Autodesk Inventor part; units mm, degrees
ref_plane "YZ Plane" through (0, 0, 0) normal (1, 0, 0) x (0, 1, 0)
ref_plane "XZ Plane" through (0, 0, 0) normal (0, 1, 0) x (-1, 0, 0)
ref_plane "XY Plane" through (0, 0, 0) normal (0, 0, 1) x (1, 0, 0)
sketch "スケッチ1" plane through (0, 0, 0) normal (0, 1, 0) x (-1, 0, 0)
  circle A0 centre (0, 0) radius 178.1675
  circle A1 centre (0, 0) radius 157.8276
  line L0 (168.1877, 0) -> (166.7488, -21.9529)
  line L1 (168.1877, 0) -> (130.1721, 2.4917) construction
  line L2 (249.4344, 0) -> (-249.4344, 0)
  line L3 (166.7488, -21.9529) -> (156.7702, -21.2989)
  line L4 (156.7702, -21.2989) -> (158.2091, 0.654) construction
  line L5 (158.2091, 0.654) -> (168.1877, 0)
  line L6 (157.4896, -10.3224) -> (0, 0)
  line L7 (166.7488, -21.9529) -> (162.4568, -43.5302)
  line L8 (162.4568, -43.5302) -> (152.649, -41.5793) construction
  line L9 (152.649, -41.5793) -> (156.9409, -20.002) construction
  line L10 (156.9409, -20.002) -> (166.7488, -21.9529) construction
  line L11 (162.4568, -43.5302) -> (155.3851, -64.3626)
  line L12 (155.3851, -64.3626) -> (145.9158, -61.1482) construction
  line L13 (145.9158, -61.1482) -> (152.9875, -40.3158) construction
  line L14 (152.9875, -40.3158) -> (162.4568, -43.5302) construction
  line L15 (155.3851, -64.3626) -> (145.6548, -84.0938)
  line L16 (145.6548, -84.0938) -> (136.6861, -79.6709) construction
  line L17 (136.6861, -79.6709) -> (146.4164, -59.9397) construction
  line L18 (146.4164, -59.9397) -> (155.3851, -64.3626) construction
  line L19 (0, 0) -> (111.6009, -111.6009)
  line L20 (145.6548, -84.0938) -> (137.3401, -78.5381) construction
  line L21 (137.3401, -78.5381) -> (125.1176, -96.8305) construction
  line L22 (125.1176, -96.8305) -> (133.4323, -102.3862) construction
  line L23 (133.4323, -102.3862) -> (145.6548, -84.0938)
  line L24 (133.4323, -102.3862) -> (125.9139, -95.7927) construction
  line L25 (125.9139, -95.7927) -> (111.4082, -112.3332) construction
  line L26 (111.4082, -112.3332) -> (118.9266, -118.9266)
  line L27 (118.9266, -118.9266) -> (133.4323, -102.3862)
  line L28 (111.6009, -111.6009) -> (118.9266, -118.9266)
  line L29 (166.7488, -21.9529) -> (176.7274, -22.6069) construction
  line L30 (118.9266, -118.9266) -> (125.9834, -125.9834)
  point P0 (154.795, -30.7906)
  point P1 (149.4517, -50.732)
  point P2 (141.5512, -69.8053)
  point P3 (131.2288, -87.6843)
  point P4 (118.661, -104.0629)
  point P5 (157.8276, 0)
  point P6 (178.1675, 0)
  dimension "d0" = 22
  dimension "d1" = 10
  dimension "d2" = 45
  dimension "d4" = 315.6551
extrude "押し出し1" add sketch "スケッチ1" along normal blind 5.5 contours L30 L27 L23 L15 L11 L7 L0 L2 A0 | L28 A1 L2 L0 L7 L11 L15 L23 L27
sketch "スケッチ2" plane through (0, 5.5, 0) normal (0, 1, 0) x (1, 0, 0)
  circle A0 centre (0, 0) radius 309.8276
  line L0 (-168.1877, 0) -> (-166.7488, 21.9529)
  line L1 (-166.7488, 21.9529) -> (-162.4568, 43.5302)
  line L2 (-162.4568, 43.5302) -> (-155.3851, 64.3626)
  line L3 (-155.3851, 64.3626) -> (-145.6548, 84.0938)
  line L4 (-133.4323, 102.3862) -> (-145.6548, 84.0938)
  line L5 (-118.9266, 118.9266) -> (-133.4323, 102.3862)
  line L6 (-167.4682, 10.9764) -> (-166.0294, 32.9293)
  line L7 (-166.0294, 32.9293) -> (-275.7938, 40.1237)
  line L8 (-275.7938, 40.1237) -> (-277.2327, 18.1708)
  line L9 (-277.2327, 18.1708) -> (-167.4682, 10.9764)
  line L10 (-164.6028, 32.7415) -> (-160.3108, 54.3188)
  line L11 (-160.3108, 54.3188) -> (-268.1972, 75.7787)
  line L12 (-268.1972, 75.7787) -> (-272.4892, 54.2015)
  line L13 (-272.4892, 54.2015) -> (-164.6028, 32.7415)
  circle A1 centre (-166.7488, 21.9529) radius 11
  circle A2 centre (-162.4568, 43.5302) radius 11
  line L14 (-158.921, 53.9464) -> (-151.8493, 74.7789)
  line L15 (-151.8493, 74.7789) -> (-256.0116, 110.1372)
  line L16 (-256.0116, 110.1372) -> (-263.0833, 89.3047)
  line L17 (-263.0833, 89.3047) -> (-158.921, 53.9464)
  circle A3 centre (-155.3851, 64.3626) radius 11
  arc A4 (-275.7591, 62.4834) -> (-281.3553, 41.7349) centre (-166.7488, 21.9529) ccw
  line L18 (-178.1663, 0.654) -> (-158.2091, -0.654)
  line L19 (-158.2091, -0.654) -> (-156.7702, 21.2989)
  line L20 (-156.7702, 21.2989) -> (-176.7274, 22.6069)
  line L21 (-176.7274, 22.6069) -> (-178.1663, 0.654)
  line L22 (-177.4468, 11.6305) -> (-275.7938, 40.1237)
  line L23 (-176.7274, 22.6069) -> (-176.008, 33.5834)
  line L24 (-176.008, 33.5834) -> (-275.7591, 62.4834)
  line L25 (-275.7938, 40.1237) -> (-281.3553, 41.7349)
  circle A5 centre (0, 0) radius 137.8276
  line L26 (0, 0) -> (-219.0812, 219.0812)
  line L27 (-111.6009, 111.6009) -> (-125.9834, 125.9834)
  line L28 (-433.7586, 0) -> (433.7586, 0)
  circle A6 centre (0, 0) radius 279.8276 construction
  arc A7 (-111.6009, 111.6009) -> (-157.8276, 0) centre (0, 0) ccw
  point P0 (-158.1662, 0)
  point P1 (-137.8276, 0)
  point P2 (-97.4588, 97.4588)
  point P3 (-309.8276, 0)
  dimension "d7" = 22
  dimension "d10" = 20
  dimension "d11" = 100
  dimension "d12" = 30
  dimension "d14" = 20
  dimension "d17" = 122
extrude "押し出し2" add sketch "スケッチ2" against normal blind 5.5 contours L26 L5 L4 L3 A3 L15 L16 L17 A2 L11 L12 L24 A4 L25 L8 L9 L21 L18 L28 A0 | L18 L21 L9 L0 | L0 A1 L19 L28 | A5 L28 A7 A1 A2 A3 L26 | L26 A7 A3 L3 L4 L5 | A1 L21 L20 L0 | L9 L21 A1 | L0 L20 L19 A1 | L19 A7 L28 | L6 A1 L1 | L20 L23 A1 L6 | L1 A1 A7 L19 L20 | L22 L7 L23 A1 L21 | L9 L8 L22 | A1 L23 L21 | A1 A7 L19 | A7 A3 L2 L3 | A3 A7 | A2 L10 L1 | A1 L7 L24 L13 | A2 A7 A1 | L13 L24 L12 L11 A2 | L1 L2 A2 A7 | A1 L23 L7 | L25 A4 L24 L12 L13 L7 | A7 A1 | A7 A2 A3 | L3 L14 A3 | L10 A2 L2 | L13 L12 L24 | A7 A2 | A3 L14 L2 | L17 L16 L15 A3
sketch "スケッチ3" plane through (0, 5.5, 0) normal (0, 1, 0) x (1, 0, 0)
  circle A0 centre (0, 0) radius 157.8276
  arc A1 (-97.4588, 97.4588) -> (-137.8276, 0) centre (0, 0) ccw
  line L0 (-97.4588, 97.4588) -> (-219.0812, 219.0812)
  line L1 (-309.8276, 0) -> (-137.8276, 0)
  arc A2 (-219.0812, 219.0812) -> (-309.8276, 0) centre (0, 0) ccw
  point P0 (-157.8276, 0)
  point P1 (-111.6009, 111.6009)
  dimension "d18" = 20
extrude "押し出し3" cut sketch "スケッチ3" against normal through all contours A0 L1 A2 L0
sketch "スケッチ4" plane through (0, 5.5, 0) normal (0, 1, 0) x (1, 0, 0)
  arc A0 (-111.6009, 111.6009) -> (-157.8276, 0) centre (0, 0) ccw
  line L0 (-157.8276, 0) -> (-137.8276, 0)
  line L1 (-137.8276, 0) -> (-137.8276, 25)
  line L2 (-137.8276, 25) -> (-157.8276, 25)
  line L3 (-157.8276, 25) -> (-157.8276, 0)
  arc A1 (-97.4588, 97.4588) -> (-137.8276, 0) centre (0, 0) ccw
  line L4 (-97.4588, 97.4588) -> (-111.6009, 111.6009)
  line L5 (-111.6009, 111.6009) -> (-129.2786, 93.9233)
  line L6 (-129.2786, 93.9233) -> (-115.1365, 79.7811)
  line L7 (-115.1365, 79.7811) -> (-97.4588, 97.4588)
  dimension "d21" = 25
  dimension "d22" = 25
extrude "押し出し4" cut sketch "スケッチ4" against normal through all contours L4 L7 L6 A0 | A0 L6 L5 | L2 L1 L0 A0 | A0 L3 L2
fillet "フィレット1" radius 1 2 edges at (-97.4588, 2.75, -97.4588) (-137.8276, 2.75, 0)
sketch "スケッチ5" plane through (0, 5.5, 0) normal (0, 1, 0) x (1, 0, 0)
  circle A0 centre (0, 0) radius 147.8276
  arc A1 (-127.8696, 92.5143) -> (-155.835, 25) centre (0, 0) ccw
  arc A2 (-137.8276, 23.48) -> (-135.842, 23.3109) centre (-136.8276, 23.48) ccw
  arc A3 (-112.5381, 79.5715) -> (-135.842, 23.3109) centre (0, 0) ccw
  arc A4 (-112.5381, 79.5715) -> (-114.0617, 80.8559) centre (-113.3546, 80.1488) ccw
  line L0 (-114.0617, 80.8559) -> (-115.1365, 79.7811)
  line L1 (-115.1365, 79.7811) -> (-127.8696, 92.5143)
  arc A5 (-127.8696, 92.5143) -> (-155.835, 25) centre (0, 0) ccw
  line L2 (-155.835, 25) -> (-137.8276, 25)
  line L3 (-137.8276, 25) -> (-137.8276, 23.48)
  point P0 (-120.7019, 85.3466)
  point P1 (-145.6983, 25)
  dimension "d26" = 10
extrude "押し出し5" cut sketch "スケッチ5" against normal through all contours L1 L0 A4 A3 A2 L3 L2 A0 picked at (-137.0003, 45.2919)
equation "\"d22\" = d21"
properties part number "back_upper" material "木材 (カエデ材)"
Geometry: final body of the model. Coordinates: model frame, mm. Round coordinates to 2 decimals unless told otherwise and drop trailing zeros. Order: outer loops, then holes, each group sorted by start corner. A loop starts at its lowest first (then second) coordinate and runs counter-clockwise, first axis right, second up. Notation, with made-up numbers: (-0.5, -23.75) -> (43.5, -23.75) arc R38 cw to (43.5, 14.25) -> close; hole circle Ø9 at (-7, 43). An arc over 180 degrees is marked (long way). Put each result on its own line as item: value. Start each with the question number.
Q1. Line query: probe 1 along Z at (x, y) = (-137.5, 2.1); probe 2 along Z at (x, y) = (-123, 2); probe 3 along X at (y, z) = (2.3, -64.5). Output: solid intervals per line, ascending.
Q2. Section B-B on x = -126. Return the cut outline in (y, z), and give its area (3 significant figures).
Q3. First-contact query: pin 1 (3 mm diameter, centred on x = -125, y = 1, fed in from +Z). Flat tip, straight axial feed; report the tip coordinate or a pass-through.
Q4. Section A-A on y = 2.5. Return the cut outline in (x, z), and give its area (3 significant figures).
Ans:
1. probe 1: z = -77.48 to -54.28
1. probe 2: z = -87.64 to -82
1. probe 3: x = -144.05 to -133.01
2. outline: (0, -90.64) -> (5.5, -90.64) -> (5.5, -77.31) -> (0, -77.31) -> close
2. area: 73.3 mm2
3. pin 1: stops at z = -76.49
4. outline: (-155.84, -25) arc R157.83 ccw to (-127.87, -92.51) -> (-120.7, -85.35) arc R147.83 cw to (-145.7, -25) -> close
4. area: 698 mm2
